```python
from build123d import *

# Parameters (mm, degrees)
F0_W     = 228
F0_H     = 100
F0_W_2   = 20
F0_H_2   = 24.5810076863
F0_H_3   = 22.8189926594
F0_H_4   = 29.1644897312
F0_W_3   = 58.2984770788
F0_H_5   = 47.4000003457
F0_H_6   = 16.9355106145
F1_DEPTH = 55
F2_W     = 225.4000006914
F2_H     = 97.4000006914
F3_DEPTH = 5


with BuildPart() as f1:
    # F0 (on Top) → F1 (new body)
    with BuildSketch(Plane.XY):
        with Locations((-66.3927308619, 15.6637772918)):
            Rectangle(F0_W, F0_H)
        with Locations((-169.0927312076, -20.7457192108)):
            Rectangle(F0_W_2, F0_H_2, mode=Mode.SUBTRACT)
        Polygon((-99.494241178, -33.0362230539), (-157.7927312076, -33.0362230539), (-157.7927312076, 15.6637772918), (-99.4942541288, 15.6637772918), align=None, mode=Mode.SUBTRACT)
        with Locations((-169.0927312076, 4.254280962)):
            Rectangle(F0_W_2, F0_H_3, mode=Mode.SUBTRACT)
        with BuildLine():
            add(Edge.make_bspline(
                [(-48.9903728661, 15.6637772918), (-50.8894876917, 10.2674604802), (-66.765290357, 1.4664925702), (-40.0663002403, -32.5316685311), (-25.9607383293, -33.0362230539)],
                knots=[0.2243177363, 0.2243177363, 0.2243177363, 0.2243177363, 0.3467822733, 0.5479791111, 0.5479791111, 0.5479791111, 0.5479791111], degree=3))
            Line((-25.9607383293, -33.0362230539), (-98.194241178, -33.0362230539))
            Line((-98.194241178, -33.0362230539), (-98.1942541288, 15.6637772918))
            Line((-98.1942541288, 15.6637772918), (-48.9903728661, 15.6637772918))
        make_face(mode=Mode.SUBTRACT)
        with BuildLine():
            add(Edge.make_bspline(
                [(-21.6105978481, -32.9644661853), (-6.3706766603, -31.3032384951), (5.0973679535, -4.3926706889), (3.8858228363, 15.6637772918)],
                knots=[0.5576009666, 0.5576009666, 0.5576009666, 0.5576009666, 0.7792958229, 0.7792958229, 0.7792958229, 0.7792958229], degree=3))
            add(Edge.make_bspline(
                [(-22.597104311, -33.0362230539), (-22.2665896559, -33.0241494524), (-21.9377248021, -33.0001246607), (-21.6105978481, -32.9644661853)],
                knots=[0.5528422567, 0.5528422567, 0.5528422567, 0.5528422567, 0.5576009666, 0.5576009666, 0.5576009666, 0.5576009666], degree=3))
            add(Edge.make_bspline(
                [(-23.6153104586, -33.0362230539), (-23.2743637388, -33.0484186836), (-22.9348725199, -33.0485616256), (-22.597104311, -33.0362230539)],
                knots=[0.5479791111, 0.5479791111, 0.5479791111, 0.5479791111, 0.5528422567, 0.5528422567, 0.5528422567, 0.5528422567], degree=3))
            add(Edge.make_bspline(
                [(-24.2891701926, -32.9966958469), (-24.0639725183, -33.0149937125), (-23.839327314, -33.0282099937), (-23.6153104586, -33.0362230539)],
                knots=[0.5447838124, 0.5447838124, 0.5447838124, 0.5447838124, 0.5479791111, 0.5479791111, 0.5479791111, 0.5479791111], degree=3))
            add(Edge.make_bspline(
                [(-46.6449449953, 15.6637772918), (-48.5440598209, 10.2674604802), (-64.2631309923, 1.5533788133), (-38.243886485, -31.8628407834), (-24.2891701926, -32.9966958469)],
                knots=[0.2243177363, 0.2243177363, 0.2243177363, 0.2243177363, 0.3467822733, 0.5447838124, 0.5447838124, 0.5447838124, 0.5447838124], degree=3))
            add(Edge.make_bspline(
                [(-46.2810248137, 16.9637772918), (-46.3742506197, 16.5161489966), (-46.4971600312, 16.0837068693), (-46.6449449953, 15.6637772918)],
                knots=[0.2147878138, 0.2147878138, 0.2147878138, 0.2147878138, 0.2243177363, 0.2243177363, 0.2243177363, 0.2243177363], degree=3))
            add(Edge.make_bspline(
                [(-61.7832280695, 64.3637776375), (-57.1571978586, 44.8554591392), (-44.1798779302, 27.0525374476), (-46.2810248137, 16.9637772918)],
                knots=[0, 0, 0, 0, 0.2147878138, 0.2147878138, 0.2147878138, 0.2147878138], degree=3))
            Line((-61.7832280695, 64.3637776375), (-58.7569419295, 64.3637776375))
            Line((-58.7569419295, 64.3637776375), (-18.4832829982, 64.3637776375))
            Line((-18.4832829982, 64.3637776375), (-16.1378551275, 64.3637776375))
            add(Edge.make_bspline(
                [(3.7889127405, 16.9637772918), (2.0816215591, 36.2077970929), (-11.2032608143, 49.1446081038), (-16.1378551275, 64.3637776375)],
                knots=[0.7841212321, 0.7841212321, 0.7841212321, 0.7841212321, 1, 1, 1, 1], degree=3))
            add(Edge.make_bspline(
                [(3.8858228363, 15.6637772918), (3.8594523508, 16.1003258471), (3.8270748012, 16.5336272046), (3.7889127405, 16.9637772918)],
                knots=[0.7792958229, 0.7792958229, 0.7792958229, 0.7792958229, 0.7841212321, 0.7841212321, 0.7841212321, 0.7841212321], degree=3))
        make_face(mode=Mode.SUBTRACT)
        with BuildLine():
            add(Edge.make_bspline(
                [(-19.5708181709, -33.0362230539), (-3.8425589006, -32.4616744452), (8.1496600722, -4.8231850372), (6.9121089764, 15.6637772918)],
                knots=[0.5528422567, 0.5528422567, 0.5528422567, 0.5528422567, 0.7792958229, 0.7792958229, 0.7792958229, 0.7792958229], degree=3))
            Line((6.9121089764, 15.6637772918), (46.3072694838, 15.6637772918))
            Line((46.3072694838, 15.6637772918), (46.3072694838, -33.0362230539))
            Line((46.3072694838, -33.0362230539), (-19.5708181709, -33.0362230539))
        make_face(mode=Mode.SUBTRACT)
        with Locations((-169.0927312076, 31.5460221574)):
            Rectangle(F0_W_2, F0_H_4, mode=Mode.SUBTRACT)
        with Locations((-128.6434926682, 40.6637774646)):
            Rectangle(F0_W_3, F0_H_5, mode=Mode.SUBTRACT)
        with Locations((-169.0927312076, 55.8960223302)):
            Rectangle(F0_W_2, F0_H_6, mode=Mode.SUBTRACT)
        with BuildLine():
            add(Edge.make_bspline(
                [(-64.1286559403, 64.3637776375), (-59.5026257294, 44.8554591392), (-46.525305801, 27.0525374476), (-48.6264526844, 16.9637772918)],
                knots=[0, 0, 0, 0, 0.2147878138, 0.2147878138, 0.2147878138, 0.2147878138], degree=3))
            Line((-48.6264526844, 16.9637772918), (-98.1942541288, 16.9637772918))
            Line((-98.1942541288, 16.9637772918), (-98.1942541288, 64.3637776375))
            Line((-98.1942541288, 64.3637776375), (-64.1286559403, 64.3637776375))
        make_face(mode=Mode.SUBTRACT)
        with BuildLine():
            Line((-13.1115689874, 64.3637776375), (46.3072694838, 64.3637776375))
            Line((46.3072694838, 64.3637776375), (46.3072694838, 16.9637772918))
            Line((46.3072694838, 16.9637772918), (6.8151988806, 16.9637772918))
            add(Edge.make_bspline(
                [(6.8151988806, 16.9637772918), (5.1079076992, 36.2077970929), (-8.1769746743, 49.1446081038), (-13.1115689874, 64.3637776375)],
                knots=[0.7841212321, 0.7841212321, 0.7841212321, 0.7841212321, 1, 1, 1, 1], degree=3))
        make_face(mode=Mode.SUBTRACT)
        with BuildLine():
            Line((1.5403949656, 15.6637772918), (3.8858228363, 15.6637772918))
            add(Edge.make_bspline(
                [(3.8858228363, 15.6637772918), (3.8594523508, 16.1003258471), (3.8270748012, 16.5336272046), (3.7889127405, 16.9637772918)],
                knots=[0.7792958229, 0.7792958229, 0.7792958229, 0.7792958229, 0.7841212321, 0.7841212321, 0.7841212321, 0.7841212321], degree=3))
            Line((3.7889127405, 16.9637772918), (1.4434848698, 16.9637772918))
            add(Edge.make_bspline(
                [(1.5403949656, 15.6637772918), (1.5140244801, 16.1003258471), (1.4816469304, 16.5336272046), (1.4434848698, 16.9637772918)],
                knots=[0.7792958229, 0.7792958229, 0.7792958229, 0.7792958229, 0.7841212321, 0.7841212321, 0.7841212321, 0.7841212321], degree=3))
        make_face()
        with BuildLine():
            Line((-43.6186588553, 15.6637772918), (1.5403949656, 15.6637772918))
            add(Edge.make_bspline(
                [(1.5403949656, 15.6637772918), (1.5140244801, 16.1003258471), (1.4816469304, 16.5336272046), (1.4434848698, 16.9637772918)],
                knots=[0.7792958229, 0.7792958229, 0.7792958229, 0.7792958229, 0.7841212321, 0.7841212321, 0.7841212321, 0.7841212321], degree=3))
            Line((1.4434848698, 16.9637772918), (-43.2547386736, 16.9637772918))
            add(Edge.make_bspline(
                [(-43.2547386736, 16.9637772918), (-43.3479644796, 16.5161489966), (-43.4708738911, 16.0837068693), (-43.6186588553, 15.6637772918)],
                knots=[0.2147878138, 0.2147878138, 0.2147878138, 0.2147878138, 0.2243177363, 0.2243177363, 0.2243177363, 0.2243177363], degree=3))
        make_face()
        with BuildLine():
            Line((-46.6449449953, 15.6637772918), (-43.6186588553, 15.6637772918))
            add(Edge.make_bspline(
                [(-43.2547386736, 16.9637772918), (-43.3479644796, 16.5161489966), (-43.4708738911, 16.0837068693), (-43.6186588553, 15.6637772918)],
                knots=[0.2147878138, 0.2147878138, 0.2147878138, 0.2147878138, 0.2243177363, 0.2243177363, 0.2243177363, 0.2243177363], degree=3))
            Line((-43.2547386736, 16.9637772918), (-46.2810248137, 16.9637772918))
            add(Edge.make_bspline(
                [(-46.2810248137, 16.9637772918), (-46.3742506197, 16.5161489966), (-46.4971600312, 16.0837068693), (-46.6449449953, 15.6637772918)],
                knots=[0.2147878138, 0.2147878138, 0.2147878138, 0.2147878138, 0.2243177363, 0.2243177363, 0.2243177363, 0.2243177363], degree=3))
        make_face()
    extrude(amount=F1_DEPTH)

    # F2 (on face) → F3 (cut)
    with BuildSketch(Plane.XY.offset(55)):
        with Locations((-66.3927308619, 15.6637772918)):
            Rectangle(F2_W, F2_H)
    extrude(amount=-F3_DEPTH, mode=Mode.SUBTRACT)


solid = f1.part
```
Model file for the job. Use its own axes, mm. A direction names the side the tool comes from. Coordinates: 2 decimals unless noted, no trailing zeros. Order: outer loops, then holes, each group sorted by start corner. A loop starts at its lowest first (then second) coordinate and runs counter-clockwise, first axis right, second up. Notation, with made-up numbers: (-2.75, 81.25) - (56.25, 81.25) arc R22 cw to (56.25, 119.25) - close; hole circle Ø1 at (-32.5, -32). An arc over 180 degrees is marked (long way). Return JSON: item names as keys, results as strings. Group by question number.
1) Saw through at B-B, the plane z = 29.5. Count the separate pieces of the cut face and the enclosed holes in it, plus the area to 3 significant figures.
2) Mould opens along Y. For faces 3 (the flat face through (46.307, 27, 27)), 4 (the flat face through (-50, 16, 0)), 5 (the flat face through (-68, 65.664, 27)) say: released by +Y, released by -Y, zero draft, split by the parting line, or undercut.
3) Tool access for faces 1 (the flat face through (-92, 16, 50)), 2 (the flat face through (-169, 47.428, 25)): list every direction of +Z, -Z, +X, -X, +Y, -Y with a clear straight run to the whole face (end or side of a thin tool).
4) Probe line 1 (Y direction, x = -155, z = 34.5); line 2 (X direction, y = -23.5, z = 19); line 3 (Y direction, x = -165, z = 29.5). List the from-to ranges inside material, lowest first. Write a range as from..to.
5) Saw through at A-A, the plane x = 25. Write the cut outline in (y, z), plus the area to 3 significant figures.
Values found:
{
 "1": {"separate pieces": "1", "enclosed holes": "12", "area": "1,960 mm²"},
 "2": {"face 3": "undercut", "face 4": "zero draft", "face 5": "released by +Y"},
 "3": {"face 1": "+Z", "face 2": "+Z, -Z"},
 "4": {"line 1": "y = -34.34..-33.04, 15.66..16.96, 64.36..65.66", "line 2": "x = -180.39..-179.09, -159.09..-157.79, -99.49..-98.19, -43.89..-41.54, -7.51..-4.49, 46.31..47.61", "line 3": "y = -34.34..-33.04, -8.46..-7.16, 15.66..16.96, 46.13..47.43, 64.36..65.66"},
 "5": {"outline": "(-34.34, 0) - (-33.04, 0) - (-33.04, 55) - (-34.34, 55) - close; (15.66, 0) - (16.96, 0) - (16.96, 50) - (15.66, 50) - close; (64.36, 0) - (65.66, 0) - (65.66, 55) - (64.36, 55) - close", "area": "208 mm²"}
}
